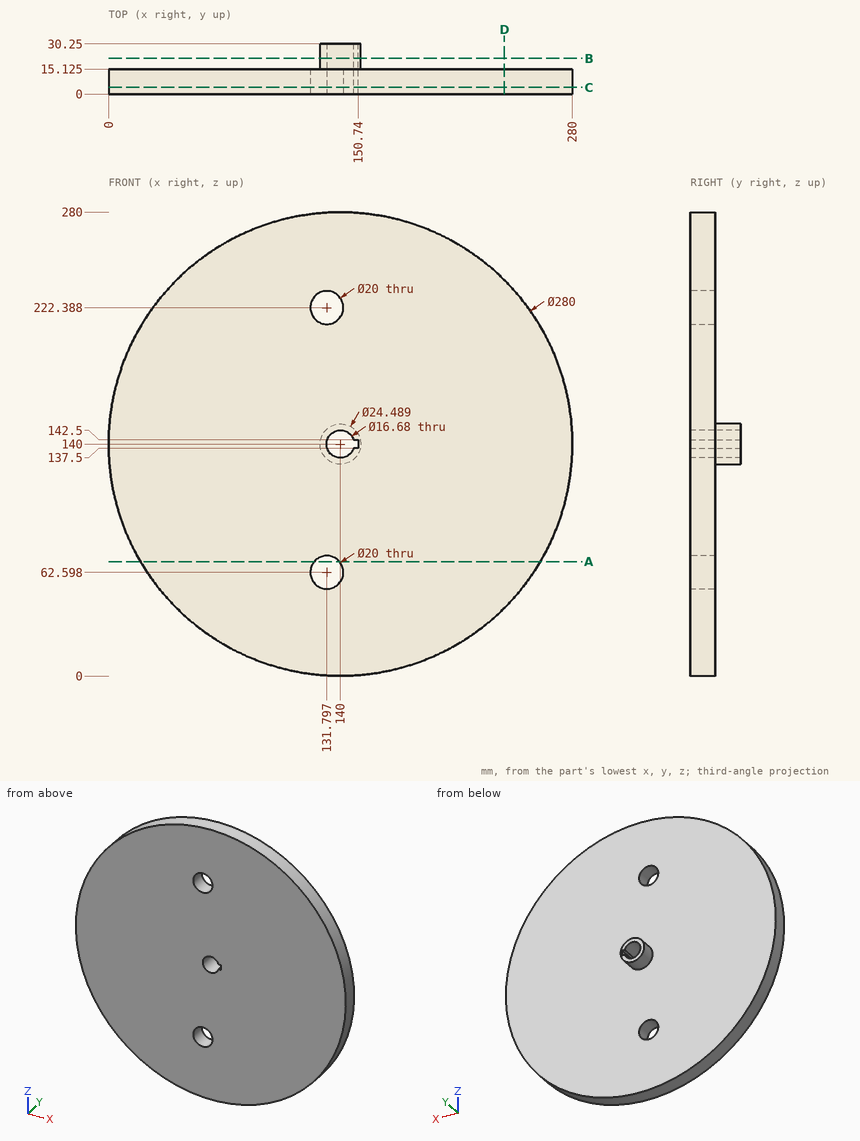
Source: three-view drawing plus pictorial views. Frame: mm from the lowest corner of the part. Round coordinates to 2 decimals unless told otherwise and drop trailing zeros. Write each loop counter-clockwise with the first axis right and the second up, starting at its lowest first coordinate (ties: lowest second). Pieces come first, ordered by that corner, then holes. Notation, with made-up numbers: M -15,-26.5 L 4,-26.5 A22 ccw 4,-5.5 Z; hole C 14,64.5 d3. An arc over 180 degrees is marked long. One line per item, written item: value. Start each with the question number.
Item 1: Section query C-C (y = 4). Return the cut outline in (x, z), plus the area to 3 significant figures.
Item 2: Section query A-A (z = 69). Return the cut outline in (x, y) (1 decimal).
Item 3: Ray query, L1, parallel to X at y = 12, z = 140; L2, parallel to Z at x = 140, y = 15 (1 decimal); L3, parallel to Y at x = 261.5, z = 95.5 (1 decimal). Return the intervals inside material, ascending. Write a range as from..to.
Item 4: Section query B-B (y = 21.5). Return the cut outline in (x, z) (1 decimal), plus the area to 3 significant figures.
Item 5: Pin query (flat end, axial travel): pin 1 (1.4 mm diameter, centred on x = 150, y = 18, fed in from -Z) (1 decimal); pin 2 (8 mm diameter, centred on y = 17.5, z = 197.5, fed in from -X); pin 3 (8 mm diameter, centred on y = 14.5, z = 219, fed in from +X) (1 decimal). Return the tip coordinate at first contact, or that it passes through.
Item 6: Section query D-D (x = 239). Return the cut outline in (y, z) (1 decimal).
Result set:
1. outline: C 140,140 d280; hole C 131.8,62.6 d20; hole C 131.8,222.39 d20; hole M 147.96,137.5 L 150.74,137.5 L 150.74,142.5 L 147.96,142.5 A8.34 ccw long Z
1. area: 60,700 mm²
2. outline: M 19.3,0 L 124.1,0 L 124.1,15.1 L 19.3,15.1 Z; M 139.5,0 L 260.7,0 L 260.7,15.1 L 139.5,15.1 Z
3. L1: x = 0..131.66, 150.74..280
3. L2: z = 0..56.9, 68.3..131.7, 148.3..216.7, 228.1..280
3. L3: y = 0..15.1
4. outline: C 140,140 d24.5; hole M 148,137.5 L 150.7,137.5 L 150.7,142.5 L 148,142.5 A8.3 ccw long Z
4. area: 240 mm²
5. pin 1: stops at z = 132
5. pin 2: stops at x = 10.95
5. pin 3: stops at x = 258.2
6. outline: M 0,41 L 15.1,41 L 15.1,239 L 0,239 Z
